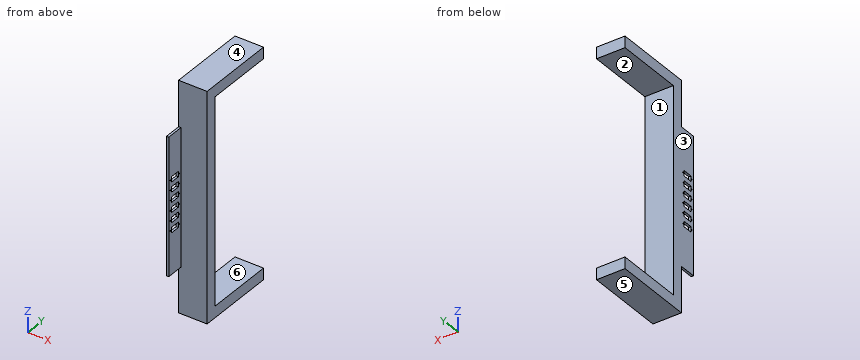
Autodesk Inventor part; units mm, degrees
ref_plane "YZ Plane" through (0, 0, 0) normal (1, 0, 0) x (0, 1, 0)
ref_plane "XZ Plane" through (0, 0, 0) normal (0, 1, 0) x (-1, 0, 0)
ref_plane "XY Plane" through (0, 0, 0) normal (0, 0, 1) x (1, 0, 0)
sketch "Sketch1" plane through (0, 0, 0) normal (0, 1, 0) x (-1, 0, 0)
  line L0 (0, 0) -> (-63.5, 0)
  line L1 (-63.5, 0) -> (-63.5, -508)
  line L2 (-63.5, -508) -> (0, -508)
  line L3 (0, -508) -> (0, 0)
  dimension "d0" = 63.5
  dimension "d1" = 508
extrude "Extrusion1" add sketch "Sketch1" along normal blind 25.4
sketch "Sketch2" plane through (0, 25.4, 0) normal (0, 1, 0) x (1, 0, 0)
  line L0 (0, 508) -> (0, 0)
  line L1 (63.5, 0) -> (63.5, 508)
  line L2 (0, 0) -> (63.5, 0)
  line L3 (63.5, 0) -> (63.5, 25.4)
  line L4 (63.5, 25.4) -> (0, 25.4)
  line L5 (0, 25.4) -> (0, 0)
  line L6 (0, 508) -> (63.5, 508)
  line L7 (63.5, 508) -> (63.5, 482.6)
  line L8 (63.5, 482.6) -> (0, 482.6)
  line L9 (0, 482.6) -> (0, 508)
  dimension "d4" = 25.4
  dimension "d5" = 25.4
extrude "Extrusion2" add sketch "Sketch2" along normal blind 152.4 contours L6 L1 L8 L0 | L4 L1 L2 L0
sketch "Sketch3" plane through (0, 0, 0) normal (0, -1, 0) x (1, 0, 0)
  line L0 (0, -482.6) -> (0, -25.4)
  line L1 (0, -406.4) -> (5.08, -406.4)
  line L2 (5.08, -406.4) -> (5.08, -101.6)
  line L3 (5.08, -101.6) -> (0, -101.6)
  line L4 (0, -101.6) -> (0, -406.4)
  point P0 (0, 0)
  dimension "d8" = 5.08
  dimension "d9" = 304.8
extrude "Extrusion3" add sketch "Sketch3" along normal blind 38.1
sketch "Sketch4" plane through (0, 0, 0) normal (-1, 0, 0) x (0, 0, 1)
  line L0 (-192.6336, -30.2006) -> (-204.6224, -30.2006)
  line L1 (-204.6224, -30.2006) -> (-204.6224, -7.8994)
  line L2 (-204.6224, -7.8994) -> (-192.6336, -7.8994)
  line L3 (-192.6336, -7.8994) -> (-192.6336, -30.2006)
  line L4 (-214.7824, -30.2006) -> (-226.7712, -30.2006)
  line L5 (-226.7712, -30.2006) -> (-226.7712, -7.8994)
  line L6 (-226.7712, -7.8994) -> (-214.7824, -7.8994)
  line L7 (-214.7824, -7.8994) -> (-214.7824, -30.2006)
  line L8 (-236.9312, -30.2006) -> (-248.92, -30.2006)
  line L9 (-248.92, -30.2006) -> (-248.92, -7.8994)
  line L10 (-248.92, -7.8994) -> (-236.9312, -7.8994)
  line L11 (-236.9312, -7.8994) -> (-236.9312, -30.2006)
  line L12 (-259.08, -30.2006) -> (-271.0688, -30.2006)
  line L13 (-271.0688, -30.2006) -> (-271.0688, -7.8994)
  line L14 (-271.0688, -7.8994) -> (-259.08, -7.8994)
  line L15 (-259.08, -7.8994) -> (-259.08, -30.2006)
  line L16 (-281.2288, -30.2006) -> (-293.2176, -30.2006)
  line L17 (-293.2176, -30.2006) -> (-293.2176, -7.8994)
  line L18 (-293.2176, -7.8994) -> (-281.2288, -7.8994)
  line L19 (-281.2288, -7.8994) -> (-281.2288, -30.2006)
  line L20 (-303.3776, -30.2006) -> (-315.3664, -30.2006)
  line L21 (-315.3664, -30.2006) -> (-315.3664, -7.8994)
  line L22 (-315.3664, -7.8994) -> (-303.3776, -7.8994)
  line L23 (-303.3776, -7.8994) -> (-303.3776, -30.2006)
  line L24 (-406.4, 0) -> (-406.4, -38.1)
  circle A0 centre (-198.628, -32.8422) radius 1.1049
  circle A1 centre (-198.628, -5.2578) radius 1.1049
  circle A2 centre (-220.7768, -32.8422) radius 1.1049
  circle A3 centre (-220.7768, -5.2578) radius 1.1049
  circle A4 centre (-242.9256, -32.8422) radius 1.1049
  circle A5 centre (-242.9256, -5.2578) radius 1.1049
  circle A6 centre (-265.0744, -32.8422) radius 1.1049
  circle A7 centre (-265.0744, -5.2578) radius 1.1049
  circle A8 centre (-287.2232, -32.8422) radius 1.1049
  circle A9 centre (-287.2232, -5.2578) radius 1.1049
  circle A10 centre (-309.372, -32.8422) radius 1.1049
  circle A11 centre (-309.372, -5.2578) radius 1.1049
  line L25 (-101.6, 0) -> (-101.6, -38.1)
  point P0 (0, 0)
  dimension "d12" = 11.9888
  dimension "d13" = 22.3012
  dimension "d14" = 11.9888
  dimension "d15" = 22.3012
  dimension "d16" = 11.9888
  dimension "d17" = 22.3012
  dimension "d18" = 11.9888
  dimension "d19" = 22.3012
  dimension "d20" = 11.9888
  dimension "d21" = 22.3012
  dimension "d22" = 11.9888
  dimension "d23" = 22.3012
  dimension "d24" = 10.16
  dimension "d25" = 10.16
  dimension "d26" = 10.16
  dimension "d27" = 10.16
  dimension "d28" = 10.16
  dimension "d29" = 91.0336
  dimension "d30" = 2.2098
  dimension "d31" = 2.2098
  dimension "d32" = 2.2098
  dimension "d33" = 2.2098
  dimension "d34" = 2.2098
  dimension "d35" = 2.2098
  dimension "d36" = 2.2098
  dimension "d37" = 2.2098
  dimension "d38" = 2.2098
  dimension "d39" = 2.2098
  dimension "d40" = 2.2098
  dimension "d41" = 2.2098
  dimension "d42" = 22.1488
  dimension "d43" = 97.028
  dimension "d44" = 22.1488
  dimension "d45" = 22.1488
  dimension "d46" = 22.1488
  dimension "d47" = 22.1488
  dimension "d48" = 22.1488
  dimension "d49" = 22.1488
  dimension "d50" = 22.1488
  dimension "d51" = 22.1488
  dimension "d52" = 22.1488
  dimension "d53" = 97.028
extrude "Extrusion4" cut sketch "Sketch4" against normal blind 5.08
properties part number "guitar bridge"
CAD build for the part. Positions are in the model's coordinates, mm. Face numbers are marked on the shaded views. A direction names the side the tool comes from. Round coordinates to 2 decimals unless told otherwise and drop trailing zeros. Order: outer loops, then holes, each group sorted by start corner. A loop starts at its lowest first (then second) coordinate and runs counter-clockwise, first axis right, second up. Notation, with made-up numbers: (3.25, -31) -> (34.25, -31) arc R17 cw to (34.25, -25) -> close; hole circle Ø7 at (-21, -26). An arc over 180 degrees is marked (long way). Write each question's results on one line, items separated by ' | '.
1. Cut at C-C (z = -182). Give the cut face in (x, y), plus the area to 3 significant figures.
Findings below:
outline: (0, -38.1) -> (5.08, -38.1) -> (5.08, 0) -> (63.5, 0) -> (63.5, 25.4) -> (0, 25.4) -> close | area: 1,810 mm²
2. 3-axis set-ups, long thin cutter, end or side, ignore diameter. For the marked faces 5 and 6: which of +Z, -Z, +X, -X, +Y, -Y reach the whole face in a straight line?
Findings below:
face 5: -Z, +X, -X, +Y, -Y | face 6: +X, -X, +Y
3. Cut at B-B (x = 13). Give the cut face in (y, z), plus the area to 3 significant figures.
Findings below:
outline: (0, -508) -> (177.8, -508) -> (177.8, -482.6) -> (25.4, -482.6) -> (25.4, -25.4) -> (177.8, -25.4) -> (177.8, 0) -> (0, 0) -> close | area: 20,600 mm²
4. Wall check: line 1 along Z through (x, y) = (56, 83.5); line 2 along Y through (x, z) = (11.5, -295); line 3 along X through (y, z) = (-2, -361.5). Give the ranges that are in metal, low to high. Write a range as [from, to].
Findings below:
line 1: z = [-508, -482.6], [-25.4, 0] | line 2: y = [0, 25.4] | line 3: x = [0, 5.08]
5. Pull direction Z, two halves, no side cores. Call the marked faces 1, 2, 3 and 4: pulls with the +Z half, pulls with the -Z half, needs draft (parallel to the pull), parting line crosses it, or undercut.
Findings below:
face 1: undercut | face 2: undercut | face 3: needs draft | face 4: pulls with the +Z half
6. Flat gauge pins, fed straight in: P1, Ø4, axis at x = 38.5, y = 19.5, coming from the +Z side; P2, Ø1.5, axis at x = 2.5, y = -22.5, coming from the -Z side; P3, Ø8, axis at x = 45, z = -392.5, coming from the -Y side; P4, Ø1.5, axis at x = 4, z = -218, coming from the +Y side. Where does each tip first touch, or does it go through?
Findings below:
P1: stops at z = 0 | P2: stops at z = -406.4 | P3: stops at y = 0 | P4: stops at y = 25.4
7. Cut at A-A (y = 136.5). Give the cut face in (x, z).
Findings below:
outline: (0, -508) -> (63.5, -508) -> (63.5, -482.6) -> (0, -482.6) -> close; (0, -25.4) -> (63.5, -25.4) -> (63.5, 0) -> (0, 0) -> close
8. Cut at D-D (z = -434.5). Give the cut face in (x, y), plus the area to 3 significant figures.
Findings below:
outline: (0, 0) -> (63.5, 0) -> (63.5, 25.4) -> (0, 25.4) -> close | area: 1,610 mm²
